from build123d import *

# Parameters (mm, degrees)
SKETCH1_R           = 8
BOSS_EXTRUDE1_DEPTH = 150
SKETCH2_W           = 40
SKETCH2_H           = 52
BOSS_EXTRUDE2_DEPTH = 20
CHAMFER1_SIZE       = 12
SKETCH3_R           = 2.5
CUT_EXTRUDE1_DEPTH  = 10
SKETCH4_W           = 80.351410155
SKETCH4_H           = 105.979847546
CUT_EXTRUDE2_DEPTH  = 41


with BuildPart() as part:
    # Sketch1 → Boss-Extrude1 (new body)
    with BuildSketch(Plane(origin=(0, 0, 0), x_dir=(0, 0, -1), z_dir=(1, 0, 0))):
        Circle(SKETCH1_R)
    extrude(amount=BOSS_EXTRUDE1_DEPTH)

    # Sketch2 → Boss-Extrude2 (add, symmetric)
    with BuildSketch(Plane(origin=(0, 0, 0), x_dir=(1, 0, 0), z_dir=(0, 1, 0))):
        with Locations((50, 0)):
            Rectangle(SKETCH2_W, SKETCH2_H)
    extrude(amount=BOSS_EXTRUDE2_DEPTH, both=True)

    # Chamfer1
    chamfer1_edges = [part.edges().sort_by_distance(p)[0] for p in [
        (50, -20, 26),
        (50, -20, -26),
    ]]
    chamfer(chamfer1_edges, length=CHAMFER1_SIZE)

    # Sketch3 → Cut-Extrude1 (cut)
    with BuildSketch(Plane(origin=(0, 20, 0), x_dir=(1, 0, 0), z_dir=(0, 1, 0))):
        with Locations((38, 20)):
            Circle(SKETCH3_R)
        with Locations((62, 20)):
            Circle(SKETCH3_R)
        with Locations((38, -20)):
            Circle(SKETCH3_R)
        with Locations((62, -20)):
            Circle(SKETCH3_R)
    extrude(amount=-CUT_EXTRUDE1_DEPTH, mode=Mode.SUBTRACT)

    # Sketch4 → Cut-Extrude2 (cut, through all)
    with BuildSketch(Plane(origin=(0, 20, 0), x_dir=(1, 0, 0), z_dir=(0, 1, 0))):
        with Locations((110.175705077, -18.887237422)):
            Rectangle(SKETCH4_W, SKETCH4_H)
    extrude(amount=-CUT_EXTRUDE2_DEPTH, mode=Mode.SUBTRACT)


solid = part.part
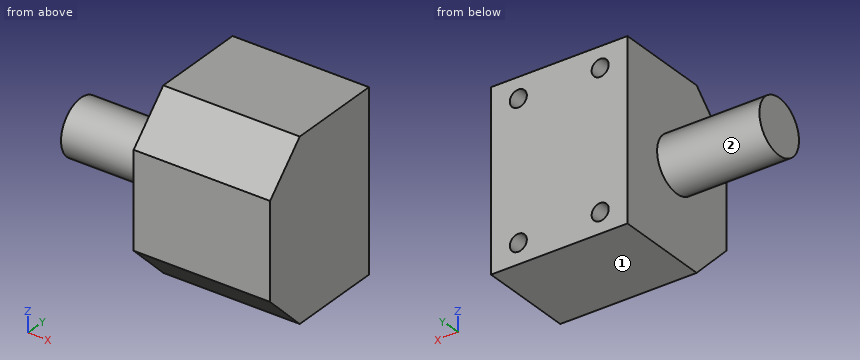
Geometry: final body of the model. Coordinates: model frame, mm. Face numbers are marked on the shaded views. A direction names the side the tool comes from. Give positions to 0.01 mm unless a question says otherwise; leave off trailing zeros. Loops run counter-clockwise (first coordinate to the right, second up) from the corner with the lowest first, then second, coordinate; pieces in that order, holes last. Notation, with made-up numbers: (39, 7.5) -> (93, 7.5) arc R24 cw to (93, 43.5) -> close; hole circle Ø1 at (76.25, -8). An arc over 180 degrees is marked (long way). Put each result on its own line as item: value.
1. Set-up query: the marked faces 1 and 2. Return all of +Z, -Z, +X, -X, +Y, -Y with unobstructed straight access to the full face (end or side cutting, diameter ignored); none if empty.
Taken from the geometry:
face 1: -Z, +X, -X, +Y, -Y
face 2: -X
2. Cut plane A-A (y = 11). Return the cut outline in (x, z).
Taken from the geometry:
outline: (30, -26) -> (70, -26) -> (70, 26) -> (30, 26) -> close; hole circle Ø5 at (38, -20); hole circle Ø5 at (38, 20); hole circle Ø5 at (62, -20); hole circle Ø5 at (62, 20)
3. Cut plane B-B (x = 62). Return the cut outline in (y, z).
Taken from the geometry:
outline: (-20, -14) -> (-8, -26) -> (20, -26) -> (20, -22.5) -> (10, -22.5) -> (10, -17.5) -> (20, -17.5) -> (20, 17.5) -> (10, 17.5) -> (10, 22.5) -> (20, 22.5) -> (20, 26) -> (-8, 26) -> (-20, 14) -> close
4. Pin query (flat end, axial travel): P1, Ø6.5, axis at x = 38, z = 20, coming from the -Y side; P2, Ø3, axis at x = 62, z = 20, coming from the -Y side; P3, Ø5.5, axis at x = 63, z = -19, coming from the +Y side; P4, Ø4, axis at x = 33.5, y = -11, coming from the +Z side. Return the tip coordinate at first contact, or that it passes through.
Taken from the geometry:
P1: stops at y = -17.25
P2: stops at y = -15.5
P3: stops at y = 20
P4: stops at z = 25
5. Ray query, line 1 along X through (y, z) = (13, 20); line 2 along Z through (x, y) = (38, 12.25); line 3 along X through (y, z) = (9.5, -2.5). Return the intervals inside material, ascending. Write a range as [from, to].
Taken from the geometry:
line 1: x = [30, 35.5], [40.5, 59.5], [64.5, 70]
line 2: z = [-26, -22.5], [-17.5, 17.5], [22.5, 26]
line 3: x = [30, 70]
6. Cut plane C-C (z = 20). Return the cut outline in (x, y), plus the area to 3 significant figures.
Taken from the geometry:
outline: (30, -14) -> (70, -14) -> (70, 20) -> (64.5, 20) -> (64.5, 10) -> (59.5, 10) -> (59.5, 20) -> (40.5, 20) -> (40.5, 10) -> (35.5, 10) -> (35.5, 20) -> (30, 20) -> close
area: 1,260 mm2
7. Cut plane D-D (y = -4). Return the cut outline in (x, z), plus the area to 3 significant figures.
Taken from the geometry:
outline: (0, -6.93) -> (30, -6.93) -> (30, -26) -> (70, -26) -> (70, 26) -> (30, 26) -> (30, 6.93) -> (0, 6.93) -> close
area: 2,500 mm2
